```python
from build123d import *

# Parameters (mm, degrees)
BOSS_EXTRUDE1_DEPTH = 20
BOSS_EXTRUDE2_DEPTH = 30
BOSS_EXTRUDE6_DEPTH = 45
CUT_EXTRUDE6_DEPTH  = 140
BOSS_EXTRUDE7_DEPTH = 25


with BuildPart() as part:
    # Sketch1 → Boss-Extrude1 (new body)
    with BuildSketch(Plane.XY):
        with BuildLine():
            Line((-68.304856892, 40.883398519), (-68.304856892, 7.883398519))
            Line((-68.304856892, 7.883398519), (-56.304856892, 7.883398519))
            Line((-56.304856892, 7.883398519), (-56.304856892, -12.116601481))
            Line((-56.304856892, -12.116601481), (-43.304856892, -12.116601481))
            Line((-43.304856892, -12.116601481), (-18.304856892, -12.116601481))
            Line((-18.304856892, -12.116601481), (-18.304856892, 10.883398519))
            ThreePointArc((-18.304856892, 10.883398519), (-39.518060328, 19.670195083), (-48.304856892, 40.883398519))
            Line((-48.304856892, 40.883398519), (-68.304856892, 40.883398519))
        make_face()
        with BuildLine():
            Line((-18.304856892, 10.883398519), (-18.304856892, -12.116601481))
            Line((-18.304856892, -12.116601481), (6.695143108, -12.116601481))
            Line((6.695143108, -12.116601481), (19.695143108, -12.116601481))
            Line((19.695143108, -12.116601481), (19.695143108, 7.883398519))
            Line((19.695143108, 7.883398519), (31.695143108, 7.883398519))
            Line((31.695143108, 7.883398519), (31.695143108, 40.883398519))
            Line((31.695143108, 40.883398519), (11.695143108, 40.883398519))
            ThreePointArc((11.695143108, 40.883398519), (2.908346543, 19.670195083), (-18.304856892, 10.883398519))
        make_face()
    extrude(amount=BOSS_EXTRUDE1_DEPTH)

    # Sketch1_3 → Boss-Extrude2 (add)
    with BuildSketch(Plane.XY):
        with BuildLine():
            Line((-38.304856892, 40.883398519), (-48.304856892, 40.883398519))
            ThreePointArc((-48.304856892, 40.883398519), (-18.304856892, 10.883398519), (11.695143108, 40.883398519))
            Line((11.695143108, 40.883398519), (1.695143108, 40.883398519))
            ThreePointArc((1.695143108, 40.883398519), (-18.304856892, 20.883398519), (-38.304856892, 40.883398519))
        make_face()
    extrude(amount=BOSS_EXTRUDE2_DEPTH)

    # Sketch1_6 → Boss-Extrude6 (add)
    with BuildSketch(Plane.XY):
        Polygon((-18.304856892, -12.116601481), (-18.304856892, -37.116601481), (31.695143108, -37.116601481), (31.695143108, 7.883398519), (19.695143108, 7.883398519), (19.695143108, -12.116601481), (6.695143108, -12.116601481), align=None)
        Polygon((-68.304856892, 7.883398519), (-68.304856892, -37.116601481), (-18.304856892, -37.116601481), (-18.304856892, -12.116601481), (-43.304856892, -12.116601481), (-56.304856892, -12.116601481), (-56.304856892, 7.883398519), align=None)
    extrude(amount=BOSS_EXTRUDE6_DEPTH)

    # Sketch3 → Cut-Extrude6 (cut)
    with BuildSketch(Plane.ZY.offset(68.304856892)):
        Polygon((45, -37.116601481), (45, -12.116601481), (20, -12.116601481), align=None)
    extrude(amount=-CUT_EXTRUDE6_DEPTH, mode=Mode.SUBTRACT)

    # Sketch3_2 → Boss-Extrude7 (add)
    with BuildSketch(Plane.ZY.offset(68.304856892)):
        Polygon((45, -37.116601481), (45, -12.116601481), (20, -12.116601481), align=None)
    boss_extrude7 = extrude(amount=-BOSS_EXTRUDE7_DEPTH)

    # Mirror1: Boss-Extrude7 across plane
    add(boss_extrude7.mirror(Plane(origin=(-18.304856892, 0, 0), x_dir=(0, 0, 1), z_dir=(1, 0, 0))))


solid = part.part
```
The model under review builds one solid part; all positions refer to its coordinate system, in mm. A direction names the side the tool comes from. Give positions to 0.01 mm unless a question says otherwise; leave off trailing zeros. Write each loop counter-clockwise with the first axis right and the second up, starting at its lowest first coordinate (ties: lowest second). Pieces come first, ordered by that corner, then holes.
(1) Consider section C-C, the plane x = -31. Give the boundary of the cut face in (y, z), and give its area (3 significant figures).
(2) Tool access review of faces 1 (the flat face through (-18.655, -24.442, 32.325)), 2 (the flat face through (19.695, -2, 32)), 3 (the flat face through (-68.305, -6, 17)), 4 (the flat face through (-19, -37.117, 22)), 5 (the flat face through (-62, 7.883, 32)): name each direction out of +Z, -Z, +X, -X, +Y, -Y from which nothing blocks a thin tool from reaching the whole face with its end or side.
(3) The part is to be moulded in two halves that separate along X. For faces 6 (the flat face through (31.695, -6, 17)), 7 (the cylindrical face through (-18.96, 10.89, 24.93)), 8 (the flat face through (13, -12.117, 33)), 9 (the flat face through (-53, 40.883, 11)), say which applies: released by +X, released by -X, zero draft, split by the parting line, or undercut.
(4) Consider section A-A, the plane y = 2.5. Give the boundary of the cut face in (x, z), and give its area (3 significant figures).
(5) For P1, Ø6, axis at y = 24, z = 27, coming from the -X side; P2, Ø10, axis at x = 15.5, y = 19, coming from the +Z side; P3, Ø4, axis at x = -23, y = 24, coming from the -Z side; P4, Ø6, axis at x = -64.5, z = 33, coming from the +Y side, all flat-tipped, find the tip position at first contact; note any pin that passes through.
(6) Consider section D-D, the plane y = 26. Give the boundary of the cut face in (x, z).
(7) To check wall thickness, follow L1, parallel to X at y = -12.5, z = 39; L2, parallel to X at y = 7, z = 37; L3, parallel to Y at x = 16.5, z = 43.5. State the ranges of each line that lie inside material, in increasing order.
(8) Consider section B-B, the plane z = 27. Give the boundary of the cut face in (x, y).
Returned:
1. outline: (-37.12, 0) - (25.43, 0) - (25.43, 30) - (13.7, 30) - (13.7, 20) - (-12.12, 20) - (-37.12, 45) - close
1. area: 1,680 mm2
2. face 1: +Z
2. face 2: +Z, +Y
2. face 3: +Z, -Z, -X, +Y, -Y
2. face 4: +Z, -Z, +X, -X, -Y
2. face 5: +Z, +X, -X, +Y
3. face 6: released by +X
3. face 7: split by the parting line
3. face 8: undercut
3. face 9: zero draft
4. outline: (-68.3, 0) - (31.7, 0) - (31.7, 45) - (19.7, 45) - (19.7, 20) - (-56.3, 20) - (-56.3, 45) - (-68.3, 45) - close
4. area: 2,600 mm2
5. P1: stops at x = -44.9
5. P2: stops at z = 20
5. P3: passes through
5. P4: stops at y = 7.88
6. outline: (-68.3, 0) - (-31.66, 0) - (-31.66, 30) - (-44.35, 30) - (-44.35, 20) - (-68.3, 20) - close; (-4.95, 0) - (31.7, 0) - (31.7, 20) - (7.74, 20) - (7.74, 30) - (-4.95, 30) - close
7. L1: x = -68.3 to -43.3, 6.7 to 31.7
7. L2: x = -68.3 to -56.3, 19.7 to 31.7
7. L3: y = -37.12 to -12.12
8. outline: (-68.3, -37.12) - (31.7, -37.12) - (31.7, 7.88) - (19.7, 7.88) - (19.7, -12.12) - (6.7, -12.12) - (6.7, -19.12) - (-43.3, -19.12) - (-43.3, -12.12) - (-56.3, -12.12) - (-56.3, 7.88) - (-68.3, 7.88) - close; (-48.3, 40.88) arc R30 ccw to (11.7, 40.88) - (1.7, 40.88) arc R20 cw to (-38.3, 40.88) - close
